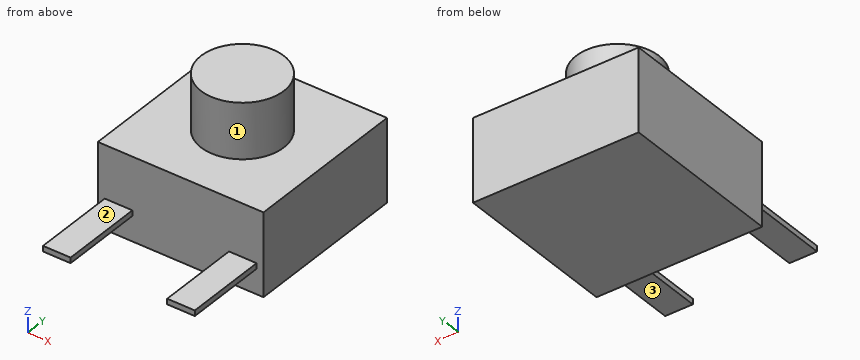
```python
from build123d import *

# Parameters (mm, degrees)
SKETCH_1_W      = 6
SKETCH_1_H      = 6
EXTRUDE_1_DEPTH = 3
SKETCH_2_R      = 1.5
EXTRUDE_2_DEPTH = 2
SKETCH_4_W      = 1
SKETCH_4_H      = 0.2


with BuildPart() as part:
    # 草图1 → 凸台-拉伸1 (new body)
    with BuildSketch(Plane.XY):
        Rectangle(SKETCH_1_W, SKETCH_1_H)
    extrude(amount=EXTRUDE_1_DEPTH)

    # 草图2 → 凸台-拉伸2 (add)
    with BuildSketch(Plane.XY.offset(3)):
        with Locations(Location((0, 0, 0), (0, 0, 180))):
            Circle(SKETCH_2_R)
    extrude(amount=EXTRUDE_2_DEPTH)

    # 扫描3: sweep along a path in 草图6
    with BuildLine(Plane(origin=(2.25, 0, 0), x_dir=(0, 0, -1), z_dir=(1, 0, 0))) as sweep_3_path:
        Line((-1.1, -3), (-1.1, -6))
    # 草图4 → 扫描3 (sweep)
    with BuildSketch(Plane.XZ.offset(3)):
        with Locations((2.25, 1)):
            Rectangle(SKETCH_4_W, SKETCH_4_H)
    sweep_3 = sweep(path=sweep_3_path.line)

    # 镜向1: 扫描3 across plane
    add(sweep_3.mirror(Plane(origin=(0, 0, 0), x_dir=(0, 0, 1), z_dir=(1, 0, 0))))


solid = part.part
```
The model under review builds one solid part; all positions refer to its coordinate system, in mm. Face numbers are marked on the shaded views. A direction names the side the tool comes from. Round coordinates to 2 decimals unless told otherwise and drop trailing zeros. Loops run counter-clockwise (first coordinate to the right, second up) from the corner with the lowest first, then second, coordinate; pieces in that order, holes last. Notation, with made-up numbers: M 6,7 L 56,7 A25 cw 56,22 Z; hole C 75.5,-31.5 d5. An arc over 180 degrees is marked long. Put each result on its own line as item: value.
Q1. For pin 1 (0.8 mm diameter, centred on x = 2, y = -4, fed in from -Z); pin 2 (2 mm diameter, centred on x = -0.5, z = 3.5, fed in from +Y); pin 3 (1.5 mm diameter, centred on x = -2, y = -2, fed in from +Z); pin 4 (0.5 mm diameter, centred on x = 2, y = -4.5, fed in from +Z), all flat-tipped, find the tip position at first contact; note any pin that passes through.
Result set:
pin 1: stops at z = 0.9
pin 2: stops at y = 3
pin 3: stops at z = 3
pin 4: stops at z = 1.1
Q2. Machinability: for the marked faces 1, 2 and 3, which of the approach directions +Z, -Z, +X, -X, +Y, -Y give a long, thin tool a straight path to every point of the face, cutting with its end or side? Answer none if there is none.
Result set:
face 1: +Z
face 2: +Z, +X, -X, -Y
face 3: -Z, +X, -X, -Y
Q3. To check wall thickness, follow L1, parallel to Z at x = -2.05, y = -1.25; L2, parallel to Y at x = -2.25, z = 0.25; L3, parallel to Y at x = -0.8, z = 3.25. State the ranges of each line that lie inside material, in increasing order.
Result set:
L1: z = 0 to 3
L2: y = -3 to 3
L3: y = -1.27 to 1.27
Q4. Consider section A-A, the plane y = 0. Give the boundary of the cut face in (x, z).
Result set:
outline: M -3,0 L 3,0 L 3,3 L 1.5,3 L 1.5,5 L -1.5,5 L -1.5,3 L -3,3 Z
Q5. Consider section D-D, the plane y = 2. Give the boundary of the cut face in (x, z).
Result set:
outline: M -3,0 L 3,0 L 3,3 L -3,3 Z
Q6. Consider section C-C, the plane z = 2.7. Give the boundary of the cut face in (x, y).
Result set:
outline: M -3,-3 L 3,-3 L 3,3 L -3,3 Z
